Read the model definition and answer for the solid it produces. Units are mm, in the model's axes. Round coordinates to 2 decimals unless told otherwise and drop trailing zeros. Write each question's results on one line, items separated by ' | '.
from build123d import *

# Parameters (mm, degrees)
F0_R     = 9.525
F0_R_2   = 6.35
F1_DEPTH = 25.4
F3_DEPTH = 15.24
F4_R     = 2.54


with BuildPart() as f1:
    # F0 (on Top) → F1 (new body)
    with BuildSketch(Plane.XY):
        with BuildLine():
            ThreePointArc((1.7145, -14.184257), (10.691786, -9.477255), (14.2875, 0))
            ThreePointArc((14.2875, 0), (10.691786, 9.477255), (1.7145, 14.184257))
            ThreePointArc((1.7145, 14.184257), (-14.2875, 0), (1.7145, -14.184257))
        make_face()
        Circle(F0_R, mode=Mode.SUBTRACT)
        with BuildLine():
            ThreePointArc((1.7145, 14.184257), (10.691786, 9.477255), (14.2875, 0))
            ThreePointArc((14.2875, 0), (10.691786, -9.477255), (1.7145, -14.184257))
            Line((1.7145, -14.184257), (40.8305, -9.456171))
            ThreePointArc((40.8305, -9.456171), (30.1625, 0), (40.8305, 9.456171))
            Line((40.8305, 9.456171), (1.7145, 14.184257))
        make_face()
        with BuildLine():
            ThreePointArc((49.2125, 0), (46.815357, 6.31817), (40.8305, 9.456171))
            ThreePointArc((40.8305, 9.456171), (30.1625, 0), (40.8305, -9.456171))
            ThreePointArc((40.8305, -9.456171), (46.815357, -6.31817), (49.2125, 0))
        make_face()
        with Locations((39.6875, 0)):
            Circle(F0_R_2, mode=Mode.SUBTRACT)
    extrude(amount=F1_DEPTH)

    # F2 (on Front) → F3 (cut, symmetric)
    with BuildSketch(Plane.XZ):
        Polygon((40.8305, 25.4), (12.7, 25.4), (40.8305, 17.862455), align=None)
        Polygon((49.2125, 25.4), (40.8305, 25.4), (40.8305, 17.862455), (49.2125, 15.616505), align=None)
    extrude(amount=F3_DEPTH, both=True, mode=Mode.SUBTRACT)

    # F4
    f4_edges = [f1.edges().sort_by_distance(p)[0] for p in [
        (26.76525, -11.156287, 21.631228),
        (-14.2875, 0, 25.4),
    ]]
    fillet(f4_edges, radius=F4_R)


solid = f1.part
Item 1: The part is cut by section A-A (z = 5). State how many separate pieces and enclosed holes the cut face has, plus the area to 3 significant figures.
Outcome:
separate pieces: 1 | enclosed holes: 2 | area: 1,000 mm2
Item 2: The mould has two halves that part along Y. Classify faces 1 (the face through (21.546, 11.787, 11.27)), 2 (the face through (-7.559, -5.796, 12.522)), 3 (the face through (20.999, -11.853, 11.27)): pulls with the +Y half, pulls with the -Y half, needs draft (parallel to the pull), parting line crosses it, or undercut.
Outcome:
face 1: pulls with the +Y half | face 2: undercut | face 3: pulls with the -Y half
Item 3: Flat-ended cylindrical pins translate along their axes: pin 1 (3 mm diameter, centred on y = -9.5, z = 12, fed in from +X); pin 2 (11.5 mm diameter, centred on x = 39.69, y = 0, fed in from -Z); pin 3 (1.5 mm diameter, centred on x = 28, z = 20, fed in from +Y); pin 4 (2 mm diameter, centred on x = 15, z = 8, fed in from -Y). Find the tip coordinate at first contact, or state that the pin passes through.
Outcome:
pin 1: stops at x = 44.86 | pin 2: passes through | pin 3: stops at y = 11.01 | pin 4: stops at y = -12.7
Item 4: Straight lines are drawn through the part: line 1 (X direction, y = -0.25, z = 10.75); line 2 (Y direction, x = 0, z = 18.25) (1 decimal); line 3 (X direction, y = 1, z = 3). For each, find the intervals that lie inside material, in ascending order.
Outcome:
line 1: x = -14.29 to -9.52, 9.52 to 33.34, 46.03 to 49.21 | line 2: y = -14.3 to -9.5, 9.5 to 14.3 | line 3: x = -14.25 to -9.47, 9.47 to 33.42, 45.96 to 49.16
